Model file for the job. Use its own axes, mm. A direction names the side the tool comes from. Round coordinates to 2 decimals unless told otherwise and drop trailing zeros. Loops run counter-clockwise (first coordinate to the right, second up) from the corner with the lowest first, then second, coordinate; pieces in that order, holes last.
from build123d import *

# Parameters (mm, degrees)
F0_W             = 46.355
F0_H             = 28.575
F1_DEPTH         = 20.955
F2_T             = -1.778
F3_R             = 2.54
F4_DEPTH         = 14.986
F5_R             = 0.889
F6_DEPTH         = 6.35
F7_R             = 3.175
F8_DEPTH         = 19.177
F8_COPIES2_COUNT = 2


# Not quite as in the source:
# - a pattern or mirror of a feature is missing from the dataset's text; its kind, count and spacing are read off the source's solid


with BuildPart() as f1:
    # F0 (on Top) → F1 (new body)
    with BuildSketch(Plane.XY):
        Rectangle(F0_W, F0_H)
    extrude(amount=F1_DEPTH)

    # F2
    f2_openings = [f1.faces().sort_by_distance(p)[0] for p in [
        (0, 0, 20.955),
    ]]
    offset(amount=F2_T, openings=f2_openings)

    # F3 (on face) → F4 (join)
    with BuildSketch(Plane.XY.offset(1.778)):
        with Locations((-11.7475, -7.62)):
            Circle(F3_R)
    f4 = extrude(amount=F4_DEPTH)

    # F4_copies: F4 across plane
    add(f4.mirror(Plane.ZX))

    # F5 (on face) → F6 (cut)
    with BuildSketch(Plane.XY.offset(16.764)):
        with Locations((-11.7475, -7.62)):
            Circle(F5_R)
    f6 = extrude(amount=-F6_DEPTH, mode=Mode.SUBTRACT)

    # F6_copies: F6 across plane
    add(f6.mirror(Plane.ZX), mode=Mode.SUBTRACT)

    # F7 (on face) → F8 (join, through all)
    with BuildSketch(Plane.XY.offset(1.778)):
        with Locations((-19.1135, -10.2235)):
            Circle(F7_R)
    f8 = extrude(amount=F8_DEPTH)

    # F8_copies: F8 across plane
    add(f8.mirror(Plane.ZX))

    # F8_copies1: F8 across plane
    add(f8.mirror(Plane(origin=(0, 0, 0), x_dir=(0, 0, 1), z_dir=(1, 0, 0))))

    # F8_copies2: F8 ×2 about axis
    f8_copies2_axis = Axis((0, 0, 0), (0, 0, 1))
    for i in range(1, F8_COPIES2_COUNT):
        add(f8.rotate(f8_copies2_axis, i * 360 / F8_COPIES2_COUNT))


solid = f1.part
Q1. Tool access for faces 1 (the face through (0, 0, 0)), 2 (the face through (0, 12.51, 11)): list every direction of +Z, -Z, +X, -X, +Y, -Y with a clear straight run to the whole face (end or side of a thin tool).
Q2. Flat gauge pins, fed straight in: P1, Ø1.4, axis at x = -11.5, y = 8, coming from the +Z side; P2, Ø8, axis at x = -11.5, y = -9.5, coming from the +Z side (3 decimals); P3, Ø1, axis at x = 2.5, y = 6.5, coming from the +Z side. Where does each tip first touch, or does it go through?
Q3. Slice it at D-D on y = 9.25. Give the cut face in (x, z) (1 decimal).
Q4. Slice it at B-B on x = 8. Give the cut face in (y, z) (1 decimal), plus the area to 3 significant figures.
Q5. Slice it at A-A on z = 3. State how many separate pieces and enclosed holes the cut face has, plus the area to 3 significant figures.
Q6. Probe line 1 (X direction, y = 2.75, z = 15.5); line 2 (Y direction, x = 0, z = 4); line 3 (X direction, y = 7.62, z = 14.25). List the from-to ranges inside material, lowest first.
Q7. Pull direction Y, two halves, no side cores. Call faces 3 (the face through (0, 14.288, 10)), 4 (the face through (0, -14.288, 10)), 5 (the face through (23.178, 0, 10)), 6 (the face through (-12.636, 7.581, 13.633)): pulls with the +Y half, pulls with the -Y half, needs draft (parallel to the pull), parting line crosses it, or undercut.
Reply:
1. face 1: -Z, +X, -X, +Y, -Y
1. face 2: +Z
2. P1: stops at z = 16.76
2. P2: stops at z = 20.955
2. P3: stops at z = 1.78
3. outline: (-23.2, 0) - (23.2, 0) - (23.2, 21) - (16.1, 21) - (16.1, 1.8) - (-9.8, 1.8) - (-9.8, 16.8) - (-13.7, 16.8) - (-13.7, 1.8) - (-16.1, 1.8) - (-16.1, 21) - (-23.2, 21) - close
4. outline: (-14.3, 0) - (14.3, 0) - (14.3, 21) - (12.5, 21) - (12.5, 1.8) - (-12.5, 1.8) - (-12.5, 21) - (-14.3, 21) - close
4. area: 119 mm2
5. separate pieces: 3
5. enclosed holes: 5
5. area: 399 mm2
6. line 1: x = -23.18 to -21.4, 21.4 to 23.18
6. line 2: y = -14.29 to -12.51, 12.51 to 14.29
6. line 3: x = -23.18 to -21.4, -20.93 to -17.3, -14.29 to -12.64, -10.86 to -9.21, 17.3 to 20.93, 21.4 to 23.18
7. face 3: pulls with the +Y half
7. face 4: pulls with the -Y half
7. face 5: needs draft
7. face 6: undercut
